Verification items for the finished model (mm, model axes). Face numbers are marked on the shaded views. A direction names the side the tool comes from. Give positions to 0.01 mm unless a question says otherwise; leave off trailing zeros. Write each loop counter-clockwise with the first axis right and the second up, starting at its lowest first coordinate (ties: lowest second). Pieces come first, ordered by that corner, then holes.
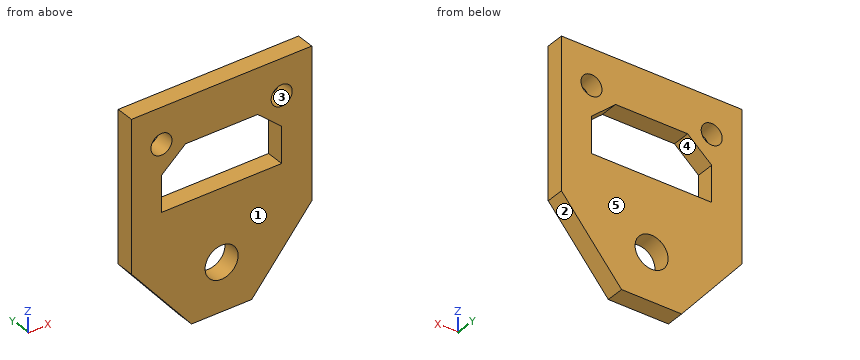
from build123d import *

# Parameters (mm, degrees)
SKETCH_2_R      = 1.75
SKETCH_2_R_2    = 2.75
EXTRUDE_2_DEPTH = 3


with BuildPart() as part:
    # 草图2 → 凸台-拉伸2 (new body)
    with BuildSketch(Plane(origin=(0, 0, 0), x_dir=(1, 0, 0), z_dir=(0, 1, 0))):
        Polygon((-15, 25), (-15, 0), (15, 0), (15, 25), (5, 37), (-5, 37), align=None)
        with Locations(Location((-10, 6, 0), (0, 0, 270))):
            Circle(SKETCH_2_R, mode=Mode.SUBTRACT)
        with Locations(Location((10, 6, 0), (0, 0, 270))):
            Circle(SKETCH_2_R, mode=Mode.SUBTRACT)
        with Locations(Location((0, 29, 0), (0, 0, 270))):
            Circle(SKETCH_2_R_2, mode=Mode.SUBTRACT)
        Polygon((-10, 17), (10, 17), (10, 11), (6, 7.5), (-6, 7.5), (-10, 11), align=None, mode=Mode.SUBTRACT)
    extrude(amount=-EXTRUDE_2_DEPTH)


solid = part.part
Item 1: Sectioned sample at A-A on z = -6. Record the cut outline in (x, y), then the cut area to 3 significant figures.
Answer key:
outline: (-15, -3) - (-11.75, -3) - (-11.75, 0) - (-15, 0) - close; (-8.25, -3) - (8.25, -3) - (8.25, 0) - (-8.25, 0) - close; (11.75, -3) - (15, -3) - (15, 0) - (11.75, 0) - close
area: 69.0 mm2
Item 2: Set-up check for the marked faces 4 and 5: record each of +Z, -Z, +X, -X, +Y, -Y from which the full face is reachable in a straight line by a thin tool's end or side.
Answer key:
face 4: +Y, -Y
face 5: +Z, -Z, +X, -X, +Y
Item 3: Scan lines: line 1 along X through (y, z) = (-1, -6); line 2 along X through (y, z) = (-2.35, -12); line 3 along Z through (x, y) = (-4.5, -1.55). Record each from-to range of solid material in increasing order.
Answer key:
line 1: x = -15 to -11.75, -8.25 to 8.25, 11.75 to 15
line 2: x = -15 to -10, 10 to 15
line 3: z = -37 to -17, -7.5 to 0
Item 4: Sectioned sample at C-C on y = -1.05. Record the cut outline in (x, z), then the cut area to 3 significant figures.
Answer key:
outline: (-15, -25) - (-5, -37) - (5, -37) - (15, -25) - (15, 0) - (-15, 0) - close; hole circle Ø3.5 at (-10, -6); hole (-10, -17) - (10, -17) - (10, -11) - (6, -7.5) - (-6, -7.5) - (-10, -11) - close; hole circle Ø5.5 at (0, -29); hole circle Ø3.5 at (10, -6)
area: 771 mm2
Item 5: Sectioned sample at D-D on x = 0. Record the cut outline in (y, z).
Answer key:
outline: (-3, -37) - (0, -37) - (0, -31.75) - (-3, -31.75) - close; (-3, -26.25) - (0, -26.25) - (0, -17) - (-3, -17) - close; (-3, -7.5) - (0, -7.5) - (0, 0) - (-3, 0) - close
Item 6: Depth check by flat-ended pin: pin 1 (5 mm diameter, centred on x = 0, z = -29, fed in from -Y); pin 2 (1.5 mm diameter, centred on x = -7.5, y = -0.5, fed in from -Z). Enter the tip coordinate at first touch or a pass-through.
Answer key:
pin 1: passes through
pin 2: stops at z = -34.9
Item 7: Release check for a two-part mould opening along X. For the marked faces 1, 2 and 3 record: released by +X, released by -X, zero draft, split by the parting line, or undercut.
Answer key:
face 1: zero draft
face 2: released by +X
face 3: undercut
Item 8: Sectioned sample at B-B on x = 3.5. Record the cut outline in (y, z), then the cut area to 3 significant figures.
Answer key:
outline: (-3, -37) - (0, -37) - (0, -17) - (-3, -17) - close; (-3, -7.5) - (0, -7.5) - (0, 0) - (-3, 0) - close
area: 82.5 mm2
